Autodesk Inventor part; units mm, degrees
ref_plane "YZ Plane" through (0, 0, 0) normal (1, 0, 0) x (0, 1, 0)
ref_plane "XZ Plane" through (0, 0, 0) normal (0, 1, 0) x (-1, 0, 0)
ref_plane "XY Plane" through (0, 0, 0) normal (0, 0, 1) x (1, 0, 0)
sketch "Sketch1" plane through (0, 0, 0) normal (0, 1, 0) x (-1, 0, 0)
  line L0 (15.4, 0) -> (-15.4, 0)
  line L1 (0, -23.8) -> (0, 23.8)
  line L2 (11, 17) -> (-11, 17)
  line L3 (-11, 17) -> (-11, -17)
  line L4 (-11, -17) -> (11, -17)
  line L5 (11, -17) -> (11, 17)
  point P0 (0, 0)
  dimension "d0" = 22
  dimension "d1" = 34
extrude "Extrusion1" add sketch "Sketch1" along normal blind 18
sketch "Sketch2" plane through (0, 18, 0) normal (0, 1, 0) x (1, 0, 0)
  line L0 (-11, -12) -> (8, -12)
  line L1 (8, -12) -> (8, 12)
  line L2 (8, 12) -> (-11, 12)
  line L3 (-11, 12) -> (-11, -12)
  line L4 (-11, -17) -> (11, -17)
  line L5 (11, -17) -> (11, 17)
  line L6 (11, 17) -> (-11, 17)
  line L7 (-11, 17) -> (-11, -17)
  line L8 (-15.4, 0) -> (15.4, 0)
  point P0 (0, 0)
  dimension "d5" = 24
  dimension "d6" = 3
extrude "Extrusion2" cut sketch "Sketch2" against normal blind 16 contours L3 L8 L1 L0 | L3 L2 L1 L8
sketch "Sketch3" plane through (-11, 0, 17) normal (0, 0, 1) x (1, 0, 0)
  line L0 (4, 18) -> (19, 18)
  line L1 (19, 18) -> (19, 2)
  line L2 (19, 2) -> (4, 2)
  line L3 (4, 2) -> (4, 18)
  line L4 (0, 18) -> (22, 18)
  line L5 (0, 0) -> (0, 18)
  line L6 (22, 0) -> (22, 18)
  line L7 (0, 0) -> (22, 0)
  point P0 (11, 0)
  dimension "d9" = 4
  dimension "d10" = 3
  dimension "d11" = 2
extrude "Extrusion3" cut sketch "Sketch3" against normal through all contours L0 L1 L2 L3
sketch "Sketch6" plane through (0, 2, 0) normal (0, 1, 0) x (1, 0, 0)
  line L0 (-11, 12) -> (-7, 12)
  line L1 (-11, -12) -> (-11, 12)
  line L2 (-7, -12) -> (-11, -12)
  line L3 (-7, -17) -> (-7, -12)
  line L4 (8, -17) -> (-7, -17)
  line L5 (-7, 17) -> (8, 17)
  line L6 (-7, 12) -> (-7, 17)
  line L7 (-15.4, 0) -> (15.4, 0)
  line L8 (0, 23.8) -> (0, -23.8)
  line L9 (8, -17) -> (8, 17)
  point P0 (0, 0)
  point P1 (0, 0)
  point P2 (0, 6)
  point P3 (0, -6)
  point P4 (-6, 0)
  dimension "d15" = 6
  dimension "d16" = 6
  dimension "d18" = 6
hole "Hole1" at (0, 2, -6) at (0, 2, 0) at (0, 2, 6) at (-6, 2, 0) direction (0, -1, 0) diameter 3 end through all
sketch "Sketch8" plane through (11, 0, 17) normal (1, 0, 0) x (0, 0, -1)
  line L0 (0, 0) -> (34, 0)
  line L1 (34, 0) -> (34, 18)
  line L2 (0, 18) -> (34, 18)
  line L3 (0, 0) -> (0, 18)
  line L4 (29, 2) -> (29, 18)
  line L5 (5, 18) -> (5, 2)
  line L6 (29, 2) -> (5, 2)
  point P0 (17, 0)
  point P1 (0, 2)
  point P2 (34, 2)
  point P3 (23.5, 12)
  point P4 (10.5, 12)
  dimension "d28" = 5.5
  dimension "d29" = 5.5
  dimension "d30" = 6
  dimension "d31" = 6
hole "Hole2" at (11, 12, -6.5) at (11, 12, 6.5) direction (-1, 0, 0) diameter 4 end through all
sketch "Sketch9" plane through (-11, 0, -17) normal (-1, 0, 0) x (0, 0, 1)
  line L0 (29, 18) -> (29, 2)
  line L1 (29, 2) -> (5, 2)
  line L2 (5, 2) -> (5, 18)
  line L3 (0, 18) -> (5, 18)
  line L4 (0, 0) -> (0, 18)
  line L5 (0, 0) -> (34, 0)
  line L6 (34, 0) -> (34, 18)
  line L7 (29, 18) -> (34, 18)
  point P0 (17, 0)
  point P1 (2.5, 12)
  point P2 (31.5, 12)
  dimension "d39" = 6
  dimension "d40" = 6
  dimension "d41" = 2.5
  dimension "d42" = 2.5
hole "Hole3" at (-11, 12, -14.5) at (-11, 12, 14.5) direction (1, 0, 0) diameter 2.5 depth 19
fillet "Fillet2" radius 1 4 edges at (-9, 18, 17) (-9, 18, -17) (-9, 18, -12) (-9, 18, 12)
fillet "Fillet4" radius 4 2 edges at (-7, 2, -14.5) (-7, 2, 14.5)
sketch "Sketch12" plane through (0, 18, 0) normal (0, 1, 0) x (1, 0, 0)
  line L0 (8, 17) -> (8, -17)
  line L1 (8, -17) -> (11, -17)
  line L2 (11, -17) -> (11, 17)
  line L3 (11, 17) -> (8, 17)
  line L4 (8, -17) -> (11, -17)
  line L5 (11, -17) -> (11, -12)
  line L6 (11, -12) -> (8, -12)
  line L7 (8, -12) -> (8, -17)
  line L8 (8, 17) -> (11, 17)
  line L9 (11, 17) -> (11, 12)
  line L10 (11, 12) -> (8, 12)
  line L11 (8, 12) -> (8, 17)
  line L12 (-11, 12) -> (-7, 12)
  line L13 (-7, -12) -> (-11, -12)
  point P0 (0, 0)
extrude "Extrusion5" cut sketch "Sketch12" against normal blind 16 contours L3 L2 L10 L0 | L6 L2 L1 L0
fillet "Fillet5" radius 4 4 edges at (9.5, 18, 12) (9.5, 18, -12) (11, 1, 17) (11, 1, -17)
fillet "Fillet6" radius 4 2 edges at (9.5, 2, -12) (9.5, 2, 12)
properties part number "bracket"
CAD build for the part. Positions are in the model's coordinates, mm. A direction names the side the tool comes from. Round coordinates to 2 decimals unless told otherwise and drop trailing zeros. Loops run counter-clockwise (first coordinate to the right, second up) from the corner with the lowest first, then second, coordinate; pieces in that order, holes last. Notation, with made-up numbers: M 35.5,12 L 82.5,12 A7 cw 82.5,23 Z; hole C 17.25,47 d1. An arc over 180 degrees is marked long. Use a Markdown table: item, result. Add a question column.
(1) Which spindle directions (+Z, -Z, +X, -X, +Y, -Y) get a long thin tool onto all of the face, cutting with end or side? Do faces 4 (the face through (-7, 10.6, 14.5)), 5 (the face through (10, 10, -12)), 6 (the face through (-9, 10, -12)), 7 (the face through (10, 10, 12)), 8 (the face through (-3, 2, 0)). Say none if no direction does.
(2) Cut at D-D (x = -6). Give the cut face in (y, z), and give its area (3 significant figures).
(3) Cut at A-A (z = 0). Give the cut face in (x, y).
(4) Drill centre lines: line 1 (X direction, y = 0.6, z = 0); line 2 (Z direction, x = 10, y = 12); line 3 (Z direction, x = 0, y = 1.5). Where is each one in solid material? Low to high.
(5) Cut at B-B (x = 0). Give the cut face in (y, z), and give its area (3 significant figures).
(6) Pull direction Y, two halves, no side cores. Call faces 1 (the face through (-5.797, 3.141, 14.465)), 2 (the face through (9.479, 10.017, -6.24)), 3 (the face through (0.9, 1, 4.8)): +Y half, -Y half, draft (parallel to the pull), parting line (faces both ways), or undercut.
(7) Flat gauge pins, fed straight in: pin 1 (3 mm diameter, centred on y = 12, z = 14.5, fed in from +X); pin 2 (3 mm diameter, centred on y = 8, z = 5, fed in from -X); pin 3 (10.5 mm diameter, centred on x = -1.5, z = 4, fed in from +Y); pin 4 (3 mm diameter, centred on y = 12, z = -6.5, fed in from +X). Where does each tip first touch, or does it go through?
(8) Cut at C-C (y = 6.75). Give the cut face in (x, z).
Geometry says:
| question | item | result |
|---|---|---|
| 1 | face 4 | +Z, -Z, +X, +Y |
| 1 | face 5 | -Z, +X, +Y |
| 1 | face 6 | -X, +Y |
| 1 | face 7 | +Z, +X, +Y |
| 1 | face 8 | +Y |
| 2 | outline | M 0,-17 L 3.35,-17 L 3.35,-12 L 2,-12 L 2,-1.5 L 0,-1.5 Z; M 0,1.5 L 2,1.5 L 2,12 L 3.35,12 L 3.35,17 L 0,17 Z |
| 2 | area | 75.5 mm² |
| 3 | outline | M -11,0 L -7.5,0 L -7.5,2 L -11,2 Z; M -4.5,0 L -1.5,0 L -1.5,2 L -4.5,2 Z; M 1.5,0 L 11,0 L 11,18 L 8,18 L 8,2 L 1.5,2 Z |
| 4 | line 1 | x = -11 to -7.5, -4.5 to -1.5, 1.5 to 11 |
| 4 | line 2 | z = -12 to -8.5, -4.5 to 4.5, 8.5 to 12 |
| 4 | line 3 | z = -17 to -7.5, -4.5 to -1.5, 1.5 to 4.5, 7.5 to 17 |
| 5 | outline | M 0,-17 L 2,-17 L 2,-7.5 L 0,-7.5 Z; M 0,-4.5 L 2,-4.5 L 2,-1.5 L 0,-1.5 Z; M 0,1.5 L 2,1.5 L 2,4.5 L 0,4.5 Z; M 0,7.5 L 2,7.5 L 2,17 L 0,17 Z |
| 5 | area | 50.0 mm² |
| 6 | face 1 | +Y half |
| 6 | face 2 | undercut |
| 6 | face 3 | draft |
| 7 | pin 1 | stops at x = -7 |
| 7 | pin 2 | stops at x = 8 |
| 7 | pin 3 | stops at y = 2 |
| 7 | pin 4 | passes through |
| 8 | outline | M -11,-17 L -7,-17 L -7,-12 L -11,-12 Z; M -11,12 L -7,12 L -7,17 L -11,17 Z; M 8,-12 L 11,-12 L 11,12 L 8,12 Z |
